For this review, take the finished solid that the model builds, in its own axes (mm). Face numbers are marked on the shaded views. A direction names the side the tool comes from. Give positions to 0.01 mm unless a question says otherwise; leave off trailing zeros. Order: outer loops, then holes, each group sorted by start corner. A loop starts at its lowest first (then second) coordinate and runs counter-clockwise, first axis right, second up.
Item 1: The part is to be moulded in two halves that separate along Z. For the marked faces 1, 2 and 3, say which applies: released by +Z, released by -Z, zero draft, split by the parting line, or undercut.
Item 2: For P1, Ø6, axis at y = 4, z = 10.5, coming from the +X side; P2, Ø14, axis at x = 138, z = 8, coming from the +Y side; P3, Ø4, axis at y = 8, z = 29.5, coming from the -X side; P4, Ø1.2, axis at x = 73.5, y = 11, coming from the -Z side, all flat-tipped, find the tip position at first contact; note any pin that passes through.
Item 3: Consider section A-A (z = 38.1). Give the boundary of the cut face in (x, y).
Item 4: Consider section C-C (y = 5.75). Give the boundary of the cut face in (x, z) (3 decimals), plus the area to 3 significant figures.
Item 5: Consider section B-B (x = 167). Give the boundary of the cut face in (y, z), plus the area to 3 significant figures.
Item 6: Machinability: for the marked faces 4 and 5, which of the approach directions +Z, -Z, +X, -X, +Y, -Y give a long, thin tool a straight path to every point of the face, cutting with its end or side? Answer none if there is none.
Item 7: Consider section D-D (z = 28). Give the boundary of the cut face in (x, y).
Item 8: For probe 1 along Z at (x, y) = (168, 1.25); probe 2 along Z at (x, y) = (82.5, 12); probe 3 along X at (y, z) = (8, 33), list the stretches that pass through material, from the lowest coordinate up.
```python
from build123d import *

# Parameters (mm, degrees)
BOSS_EXTRUDE1_DEPTH = 76.2
SKETCH2_W           = 193.548
SKETCH2_H           = 12.7
CUT_EXTRUDE1_DEPTH  = 2.3622
SKETCH3_R           = 15.875
CUT_EXTRUDE2_DEPTH  = 13.7


with BuildPart() as part:
    # Sketch1 → Boss-Extrude1 (new body)
    with BuildSketch(Plane.XY):
        Polygon((0, 0), (193.548, 0), (188.287487758, 12.7), (5.260512242, 12.7), align=None)
    extrude(amount=BOSS_EXTRUDE1_DEPTH)

    # Sketch2 → Cut-Extrude1 (cut)
    with BuildSketch(Plane(origin=(0, 12.7, 0), x_dir=(1, 0, 0), z_dir=(0, 1, 0))):
        with Locations((96.774, -6.35)):
            Rectangle(SKETCH2_W, SKETCH2_H)
    extrude(amount=-CUT_EXTRUDE1_DEPTH, mode=Mode.SUBTRACT)

    # Sketch3 → Cut-Extrude2 (cut, through all)
    with BuildSketch(Plane.XZ):
        with Locations((168.148, 38.1)):
            Circle(SKETCH3_R)
    extrude(amount=-CUT_EXTRUDE2_DEPTH, mode=Mode.SUBTRACT)


solid = part.part
```
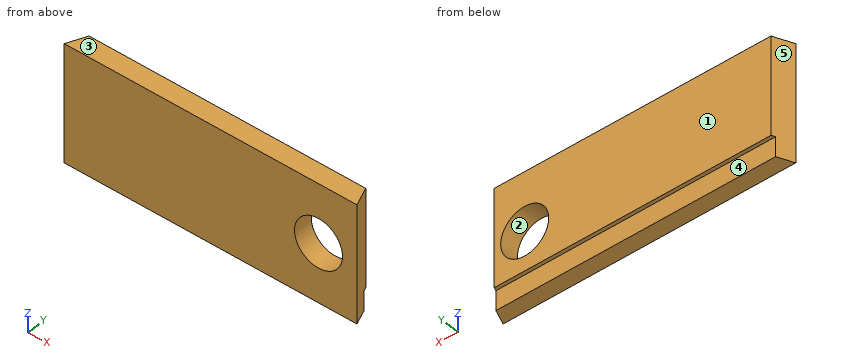
Resolved:
1. face 1: zero draft
1. face 2: undercut
1. face 3: released by +Z
2. P1: stops at x = 193.13
2. P2: stops at y = 12.7
2. P3: stops at x = 2.49
2. P4: stops at z = 12.7
3. outline: (0, 0) - (152.27, 0) - (152.27, 12.7) - (5.26, 12.7) - close; (184.02, 0) - (193.55, 0) - (188.29, 12.7) - (184.02, 12.7) - close
4. outline: (2.382, 0) - (191.166, 0) - (191.166, 76.2) - (2.382, 76.2) - close; hole circle Ø31.75 at (168.148, 38.1)
4. area: 13,600 mm2
5. outline: (0, 0) - (10.34, 0) - (10.34, 12.7) - (12.7, 12.7) - (12.7, 22.27) - (0, 22.27) - close; (0, 53.93) - (12.7, 53.93) - (12.7, 76.2) - (0, 76.2) - close
5. area: 536 mm2
6. face 4: -Z, +X, -X, +Y
6. face 5: +Z, -Z, -X, +Y
7. outline: (0, 0) - (155.9, 0) - (155.9, 12.7) - (5.26, 12.7) - close; (180.4, 0) - (193.55, 0) - (188.29, 12.7) - (180.4, 12.7) - close
8. probe 1: z = 0 to 22.23, 53.97 to 76.2
8. probe 2: z = 12.7 to 76.2
8. probe 3: x = 3.31 to 153.11, 183.18 to 190.23
